from build123d import *

# Parameters (mm, degrees)
SKETCH_R      = 24.5
PAD_DEPTH     = 10
FILLET_R      = 5
THICKNESS_T   = -1
SKETCH001_R   = 26
SKETCH001_R_2 = 23
PAD001_DEPTH  = 1


with BuildPart() as part:
    # Sketch → Pad (new body)
    with BuildSketch(Plane.XY):
        Circle(SKETCH_R)
    extrude(amount=PAD_DEPTH)

    # Fillet
    fillet_edges = [part.edges().sort_by_distance(p)[0] for p in [
        (-24.5, 0, 0),
    ]]
    fillet(fillet_edges, radius=FILLET_R)

    # Thickness
    thickness_openings = [part.faces().sort_by_distance(p)[0] for p in [
        (0, 0, 10),
    ]]
    offset(amount=THICKNESS_T, openings=thickness_openings)

    # Sketch001 → Pad001 (new body)
    with BuildSketch(Plane.XY.offset(10)):
        Circle(SKETCH001_R)
        Circle(SKETCH001_R_2, mode=Mode.SUBTRACT)
    extrude(amount=PAD001_DEPTH)


solid = part.part
Part model, mm, in its own coordinate system. A direction names the side the tool comes from. Round coordinates to 2 decimals unless told otherwise and drop trailing zeros. Write each loop counter-clockwise with the first axis right and the second up, starting at its lowest first coordinate (ties: lowest second). Pieces come first, ordered by that corner, then holes. Notation, with made-up numbers: (-9.5, 16) - (11.5, 16) arc R19 cw to (11.5, 36) - close; hole circle Ø10 at (11, -27). An arc over 180 degrees is marked (long way). Use CSV: the item, a comma, the result in double quotes.
Item 1: Tool access for faces 4 (the cylindrical face through (-2.994, 22.804, 10.493)), 5 (the cylindrical face through (22.4, 7.1, 7.5)), 6 (the flat face through (10, -21, 11)): list every direction of +Z, -Z, +X, -X, +Y, -Y with a clear straight run to the whole face (end or side of a thin tool).
Results list:
face 4,"+Z"
face 5,"none"
face 6,"+Z, +X, -X, +Y, -Y"
Item 2: Slice it at A-A, the plane x = 0. Write the cut outline in (y, z), then the cut area to 3 significant figures.
Results list:
outline,"(-26, 10) - (-24.5, 10) - (-24.5, 5) arc R5 ccw to (-19.5, 0) - (19.5, 0) arc R5 ccw to (24.5, 5) - (24.5, 10) - (26, 10) - (26, 11) - (23, 11) - (23, 10) - (23.5, 10) - (23.5, 5) arc R4 cw to (19.5, 1) - (-19.5, 1) arc R4 cw to (-23.5, 5) - (-23.5, 10) - (-23, 10) - (-23, 11) - (-26, 11) - close"
area,"69.1 mm²"
Item 3: Slice it at D-D, the plane z = 2.25. Write the cut outline in (x, y), then the cut area to 3 significant figures.
Results list:
outline,"circle Ø47.35 at (0, 0); hole circle Ø44.81 at (0, 0)"
area,"184 mm²"
Item 4: Wall check: L1, parallel to Y at x = 0, z = 6.15; L2, parallel to X at y = -0.5, z = 5.25; L3, parallel to Y at x = 0, z = 10.7. Give the ranges that are in metal, low to high.
Results list:
L1,"y = -24.5 to -23.5, 23.5 to 24.5"
L2,"x = -24.49 to -23.49, 23.49 to 24.49"
L3,"y = -26 to -23, 23 to 26"
Item 5: Slice it at B-B, the plane z = 8.5. Write the cut outline in (x, y).
Results list:
outline,"circle Ø49 at (0, 0); hole circle Ø47 at (0, 0)"
Item 6: Flat gauge pins, fed straight in: P1, Ø6, axis at x = 6.5, z = 5.5, coming from the -Y side; P2, Ø3, axis at x = -13.5, y = -3, coming from the +Z side; P3, Ø2, axis at x = 4, z = 4.5, coming from the +Y side. Where does each tip first touch, or does it go through?
Results list:
P1,"stops at y = -24.25"
P2,"stops at z = 1"
P3,"stops at y = 24.31"
Item 7: Pull direction X, two halves, no side cores. Call faces 1 (the flat face through (-17.5, 17.5, 10)), 2 (the flat face through (16, -17, 10)), 3 (the cylindrical face through (13.17, 20.66, 7.46)): pulls with the +X half, pulls with the -X half, needs draft (parallel to the pull), parting line crosses it, or undercut.
Results list:
face 1,"needs draft"
face 2,"undercut"
face 3,"parting line crosses it"
